The listing builds one solid part. Answer for the finished solid, in the listing's coordinates (mm). Face numbers are marked on the shaded views. A direction names the side the tool comes from. Coordinates: 2 decimals unless noted, no trailing zeros. Order: outer loops, then holes, each group sorted by start corner. A loop starts at its lowest first (then second) coordinate and runs counter-clockwise, first axis right, second up.
Autodesk Inventor part; units mm, degrees
ref_plane "YZ Plane" through (0, 0, 0) normal (1, 0, 0) x (0, 1, 0)
ref_plane "XZ Plane" through (0, 0, 0) normal (0, 1, 0) x (-1, 0, 0)
ref_plane "XY Plane" through (0, 0, 0) normal (0, 0, 1) x (1, 0, 0)
sketch "Sketch1" plane through (0, 0, 0) normal (0, 1, 0) x (-1, 0, 0)
  arc A0 (148.5653, -569.1641) -> (148.5653, -373.8126) centre (170, -471.4884) ccw
  arc A1 (4.7545, -533.3058) -> (4.7545, -409.6709) centre (0, -471.4884) ccw
  arc A2 (-6.2783, -274.6993) -> (-114.7972, -291.2071) centre (-60, -286.4884) ccw
  arc A3 (-114.7972, -651.7696) -> (-6.2783, -668.2775) centre (-60, -656.4884) ccw
  arc A4 (-6.2783, -274.6993) -> (148.5653, -373.8126) centre (120.7001, -246.8341) ccw
  arc A5 (148.5653, -569.1641) -> (-6.2783, -668.2775) centre (120.7001, -696.1426) ccw
  arc A6 (-114.7972, -291.2071) -> (4.7545, -409.6709) centre (14.7235, -280.0537) ccw
  arc A7 (4.7545, -533.3058) -> (-114.7972, -651.7696) centre (14.7235, -662.923) ccw
  circle A8 centre (-60, -286.4884) radius 35
  arc A9 (214.1588, -453.9884) -> (214.1588, -488.9884) centre (170, -471.4884) ccw
  circle A10 centre (-60, -656.4884) radius 35
  line L0 (232.5, -453.9884) -> (214.1588, -453.9884)
  line L1 (214.1588, -488.9884) -> (232.5, -488.9884)
  line L2 (232.5, -488.9884) -> (232.5, -453.9884)
  point P0 (0, 0)
  dimension "d0" = 200
  dimension "d1" = 124
  dimension "d2" = 170
  dimension "d3" = 110
  dimension "d4" = 110
  dimension "d5" = 370
  dimension "d6" = 185
  dimension "d7" = 260
  dimension "d8" = 230
  dimension "d9" = 0
  dimension "d10" = 260
  dimension "d11" = 0
  dimension "d12" = 260
  dimension "d13" = 260
  dimension "d14" = 70
  dimension "d15" = 70
  dimension "d16" = 95
  dimension "d17" = 35
  dimension "d18" = 17.5
  dimension "d19" = 62.5
extrude "Extrusion1" add sketch "Sketch1" along normal blind 50
equation "\"d4\" = d3"
equation "\"d6\" = 0.5 * d5"
equation "\"d10\" = d7"
equation "\"d18\" = 0.5 * d17"
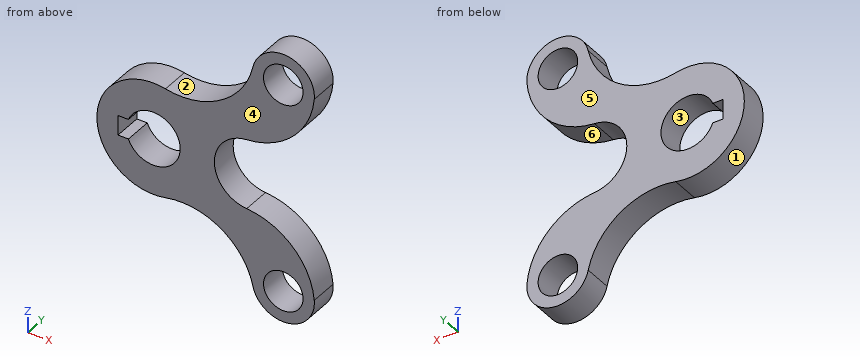
1) Straight lines are drawn through the part: probe 1 along Z at (x, y) = (-170.5, 18); probe 2 along Z at (x, y) = (60, 36); probe 3 along Z at (x, y) = (84.5, 42.5). For each, find the intervals that lie inside material, in ascending order.
2) For the marked faces 5 and 6, determine the directions among +Z, -Z, +X, -X, +Y, -Y from which every point of the face is accessible in a straight line to the end or side of a thin tool.
3) A cutting plane is placed at A-A, the plane x = -170. Write down the section's boundary in (y, z), plus the area to 3 significant figures.
4) A cutting plane is placed at D-D, the plane x = 60. Write down the section's boundary in (y, z), plus the area to 3 significant figures.
5) A cutting plane is placed at B-B, the plane z = -311.5. Write down the section's boundary in (x, y), plus the area to 3 significant figures.
6) Each of these flat-tipped pins is pushed along its axis until it touches: P1, Ø12, axis at x = -149, y = 12, coming from the -Z side; P2, Ø8, axis at y = 14.5, z = -522, coming from the +X side; P3, Ø6, axis at y = 30.5, z = -308, coming from the +X side. Where does it stop, or does it pass through?
7) The mould has two halves that part along Z. Classify the marked faces 1, 2, 3 and 4: released by +Z, released by -Z, zero draft, split by the parting line, or undercut.
8) A cutting plane is placed at C-C, the plane y = 36. Write down the section's boundary in (x, z), plus the area to 3 significant figures.
Working result:
1. probe 1: z = -571.49 to -518.99, -423.99 to -371.49
1. probe 2: z = -711.49 to -691.49, -621.49 to -556.54, -386.43 to -321.49, -251.49 to -231.49
1. probe 3: z = -705.73 to -681.48, -631.49 to -578.93, -364.05 to -311.48, -261.49 to -237.25
2. face 5: +Z, -Z, +X, -X, +Y
2. face 6: +X, +Y, -Y
3. outline: (0, -571.49) - (50, -571.49) - (50, -518.99) - (0, -518.99) - close; (0, -423.99) - (50, -423.99) - (50, -371.49) - (0, -371.49) - close
3. area: 5,250 mm2
4. outline: (0, -711.49) - (50, -711.49) - (50, -691.49) - (0, -691.49) - close; (0, -621.49) - (50, -621.49) - (50, -556.54) - (0, -556.54) - close; (0, -386.43) - (50, -386.43) - (50, -321.49) - (0, -321.49) - close; (0, -251.49) - (50, -251.49) - (50, -231.49) - (0, -231.49) - close
4. area: 8,490 mm2
5. outline: (-7.92, 0) - (35.52, 0) - (35.52, 50) - (-7.92, 50) - close; (84.48, 0) - (111.42, 0) - (111.42, 50) - (84.48, 50) - close
5. area: 3,520 mm2
6. P1: stops at z = -570.36
6. P2: stops at x = -29.54
6. P3: stops at x = 112.86
7. face 1: split by the parting line
7. face 2: released by +Z
7. face 3: undercut
7. face 4: zero draft
8. outline: (-148.57, -569.16) arc R130 cw to (6.28, -668.28) arc R55 ccw to (114.8, -651.77) arc R130 ccw to (-4.75, -533.31) arc R62 cw to (-4.75, -409.67) arc R130 ccw to (114.8, -291.21) arc R55 ccw to (6.28, -274.7) arc R130 cw to (-148.57, -373.81) arc R100 ccw (long way) to start; hole (-232.5, -488.99) - (-214.16, -488.99) arc R47.5 ccw (long way) to (-214.16, -453.99) - (-232.5, -453.99) - close; hole circle Ø70 at (60, -656.49); hole circle Ø70 at (60, -286.49)
8. area: 62,900 mm2
